Here's how the part is built. I have some questions about the finished solid (model axes, mm). Face numbers are marked on the shaded views. Coordinates: 2 decimals unless noted, no trailing zeros. Write each loop counter-clockwise with the first axis right and the second up, starting at its lowest first coordinate (ties: lowest second). Pieces come first, ordered by that corner, then holes.
Item 1: I want a section at A-A (x = 0). Please give me the cut outline in (y, z).
Item 2: Please list where these lines run through material, in increasing order: line 1 (Y direction, x = 0, z = 3.5); line 2 (X direction, y = -17.5, z = 4.75); line 3 (Z direction, x = 21, y = 3).
Item 3: I want a section at B-B (y = 0). Please give me the cut outline in (x, z).
Item 4: I'm going to push flat-ended pins straight in: P1, Ø8, axis at x = 21, y = -1, coming from the +Z side; P2, Ø10, axis at y = 13, z = 75.5, coming from the -X side; P3, Ø6, axis at x = 9.5, z = 94, coming from the +Y side. Where does each tip first touch, or does it pass through?
Item 5: I want a section at C-C (y = 17.5). Count the separate pieces of the cut face and the enclosed holes in it, and give its area (3 significant figures).
Item 6: I want a section at D-D (z = 178.5). Please give me the cut outline in (x, y), and give its area (3 significant figures).
Item 7: If we mould it in two halves opening along X, with no side actions, what happens to the marked faces 1 and 2? For each: pulls with the +X half, pulls with the -X half, needs draft (parallel to the pull), parting line crosses it, or undercut.
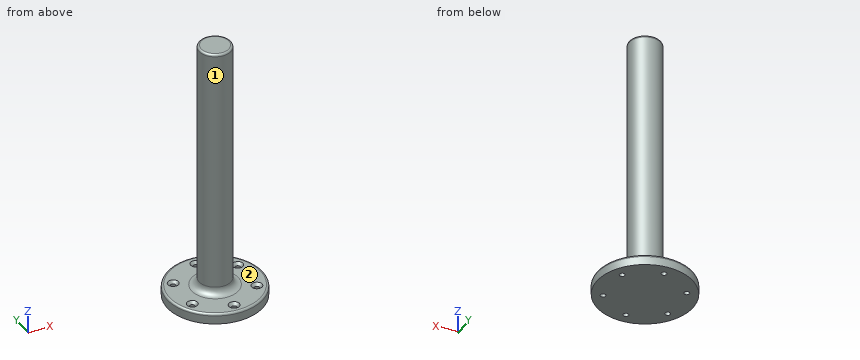
from build123d import *

# Parameters (mm, degrees)
F0_R           = 45
F1_DEPTH       = 10
F2_R           = 15
F3_DEPTH       = 250
F5_D           = 5
F5_CSINK_D     = 10
F5_CSINK_ANGLE = 90
F6_R           = 7
F7_R           = 2
F8_R           = 2


with BuildPart() as f1:
    # F0 (on Top) → F1 (new body)
    with BuildSketch(Plane.XY):
        Circle(F0_R)
    extrude(amount=F1_DEPTH)

    # F2 (on Top) → F3 (join)
    with BuildSketch(Plane.XY):
        Circle(F2_R)
    extrude(amount=F3_DEPTH)

    # F5 (through all)
    with Locations(Plane.XY.offset(10)):
        with Locations((0, 35), (-30.310889, 17.5), (-30.310889, -17.5), (0, -35), (30.310889, -17.5), (30.310889, 17.5)):
            CounterSinkHole(F5_D / 2, F5_CSINK_D / 2, counter_sink_angle=F5_CSINK_ANGLE)

    # F6
    f6_edges = [f1.edges().sort_by_distance(p)[0] for p in [
        (-15, 0, 10),
    ]]
    fillet(f6_edges, radius=F6_R)

    # F7
    f7_edges = [f1.edges().sort_by_distance(p)[0] for p in [
        (-15, 0, 250),
    ]]
    fillet(f7_edges, radius=F7_R)

    # F8
    f8_edges = [f1.edges().sort_by_distance(p)[0] for p in [
        (-45, 0, 10),
    ]]
    fillet(f8_edges, radius=F8_R)


solid = f1.part
Answer:
1. outline: (-45, 0) - (-37.5, 0) - (-37.5, 7.5) - (-40, 10) - (-43, 10) arc R2 ccw to (-45, 8) - close; (-32.5, 0) - (32.5, 0) - (32.5, 7.5) - (30, 10) - (22, 10) arc R7 cw to (15, 17) - (15, 248) arc R2 ccw to (13, 250) - (-13, 250) arc R2 ccw to (-15, 248) - (-15, 17) arc R7 cw to (-22, 10) - (-30, 10) - (-32.5, 7.5) - close; (37.5, 0) - (45, 0) - (45, 8) arc R2 ccw to (43, 10) - (40, 10) - (37.5, 7.5) - close
2. line 1: y = -45 to -37.5, -32.5 to 32.5, 37.5 to 45
2. line 2: x = -41.46 to -32.81, -27.81 to 27.81, 32.81 to 41.46
2. line 3: z = 0 to 10.04
3. outline: (-45, 0) - (45, 0) - (45, 8) arc R2 ccw to (43, 10) - (22, 10) arc R7 cw to (15, 17) - (15, 248) arc R2 ccw to (13, 250) - (-13, 250) arc R2 ccw to (-15, 248) - (-15, 17) arc R7 cw to (-22, 10) - (-43, 10) arc R2 ccw to (-45, 8) - close
4. P1: stops at z = 12.08
4. P2: stops at x = -12.69
4. P3: stops at y = 13.52
5. separate pieces: 3
5. enclosed holes: 0
5. area: 737 mm2
6. outline: circle Ø30 at (0, 0)
6. area: 707 mm2
7. face 1: parting line crosses it
7. face 2: needs draft
